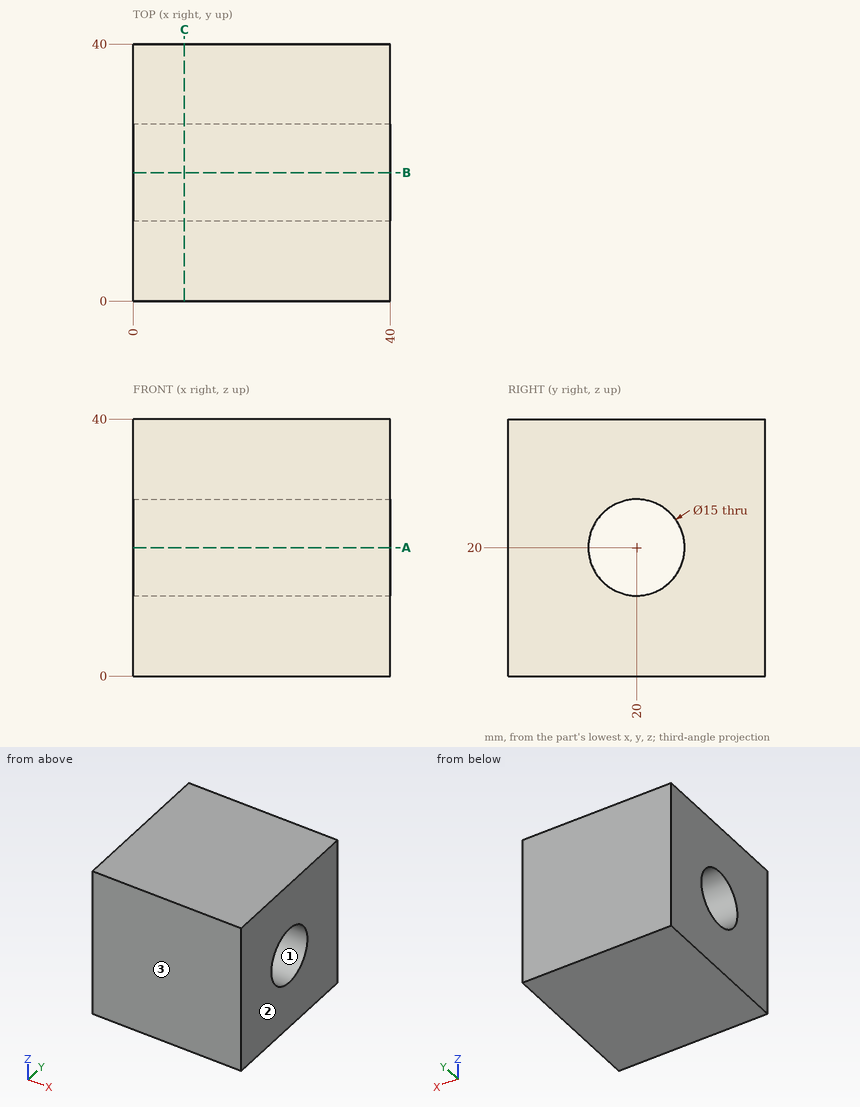
The drawing under review shows one solid part. Ordinate dimensions are in mm from its lowest x, y, z. Round coordinates to 2 decimals unless told otherwise and drop trailing zeros. Loops run counter-clockwise (first coordinate to the right, second up) from the corner with the lowest first, then second, coordinate; pieces in that order, holes last. Notation, with made-up numbers: (-35.5, -4.75) -> (18.5, -4.75) arc R18 cw to (18.5, 7.25) -> close; hole circle Ø10 at (60, 84.25). An arc over 180 degrees is marked (long way). One line per question, with ' | ' between items. Start each with the question number.
Item 1: Add section C-C, the plane x = 8. Write out the cut boundary in (y, z), then the cut area to 3 significant figures.
Item 2: Draft analysis for pull direction Y (two halves, no side actions). For the marked faces 1, 2 and 3, state which applies: +Y half, -Y half, draft (parallel to the pull), parting line (faces both ways), or undercut.
Item 3: Add section A-A, the plane z = 20. Write out the cut boundary in (x, y), then the cut area to 3 significant figures.
Item 4: Wall thickness on line 1 along Z through (x, y) = (12, 20); line 2 along Y through (x, z) = (33.5, 14); line 3 along Z through (x, y) = (15, 17): over which ranges is each line inside the solid? List them lowest first. Write a range as [from, to].
Return value:
1) outline: (0, 0) -> (40, 0) -> (40, 40) -> (0, 40) -> close; hole circle Ø15 at (20, 20) | area: 1,420 mm2
2) face 1: undercut | face 2: draft | face 3: -Y half
3) outline: (0, 0) -> (40, 0) -> (40, 12.5) -> (0, 12.5) -> close; (0, 27.5) -> (40, 27.5) -> (40, 40) -> (0, 40) -> close | area: 1,000 mm2
4) line 1: z = [0, 12.5], [27.5, 40] | line 2: y = [0, 15.5], [24.5, 40] | line 3: z = [0, 13.13], [26.87, 40]
